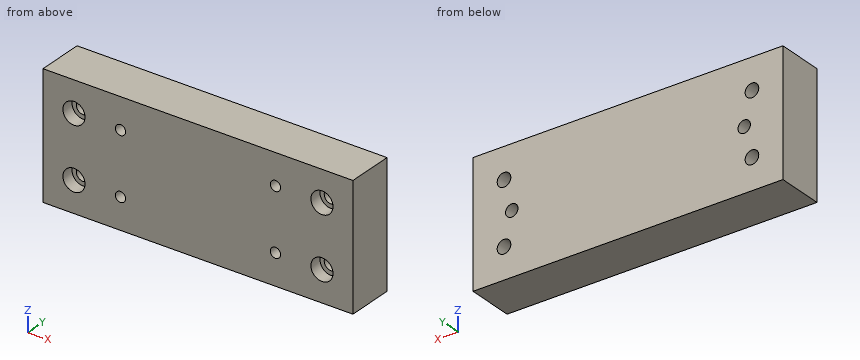
```python
from build123d import *

# Parameters (mm, degrees)
F0_W           = 200
F0_H           = 80
F1_DEPTH       = 30
F2_R           = 4
F3_DEPTH       = 10
F5_D           = 8.8
F5_CBORE_D     = 14.25
F5_CBORE_DEPTH = 8
F7_D           = 6.6
F7_DEPTH       = 12
F7_TIP         = 1.9828400428


with BuildPart() as f1:
    # F0 (on Front) → F1 (new body)
    with BuildSketch(Plane.XZ):
        Rectangle(F0_W, F0_H)
    extrude(amount=F1_DEPTH)

    # F2 (on face) → F3 (cut)
    with BuildSketch(Plane(origin=(0, 0, 0), x_dir=(-1, 0, 0), z_dir=(0, 1, 0))):
        with Locations((-75, 0)):
            Circle(F2_R)
        with Locations((75, 0)):
            Circle(F2_R)
    extrude(amount=-F3_DEPTH, mode=Mode.SUBTRACT)

    # F5 (through all)
    with Locations(Plane.XZ.offset(30)):
        with Locations((-80, 20), (-80, -20), (80, 20), (80, -20)):
            CounterBoreHole(F5_D / 2, F5_CBORE_D / 2, F5_CBORE_DEPTH)

    # F7
    with Locations(Plane.XZ.offset(30)):
        with Locations((-50, -20), (-50, 20), (50, 20), (50, -20)):
            Hole(F7_D / 2, depth=F7_DEPTH)
            with Locations((0, 0, -(F7_DEPTH + F7_TIP / 2))):  # 118° drill point
                Cone(0, F7_D / 2, F7_TIP, mode=Mode.SUBTRACT)


solid = f1.part
```
CAD build for the part. Positions are in the model's coordinates, mm. Round coordinates to 2 decimals unless told otherwise and drop trailing zeros. Order: outer loops, then holes, each group sorted by start corner. A loop starts at its lowest first (then second) coordinate and runs counter-clockwise, first axis right, second up.
Item 1: Probe line 1 along Z through (x, y) = (-80, -15.5); line 2 along Z through (x, y) = (80, -27.75) (3 decimals); line 3 along X through (y, z) = (-14, -16.5). List the from-to ranges inside material, lowest first.
Item 2: Saw through at B-B on z = 0. Write the cut outline in (x, y).
Item 3: Saw through at A-A on y = -8.25. Write the cut outline in (x, z).
Item 4: Pin check, flat tips, straight feed: pin 1 (4.5 mm diameter, centred on x = 79.5, z = -18.5, fed in from -Y) (1 decimal); pin 2 (4 mm diameter, centred on x = 76.5, z = 0.5, fed in from +Y); pin 3 (4.5 mm diameter, centred on x = -79.5, z = 23, fed in from -Y); pin 4 (5.5 mm diameter, centred on x = 50, z = 20, fed in from -Y). Stop position of each tip, or through.
Reported:
1. line 1: z = -40 to -24.4, -15.6 to 15.6, 24.4 to 40
1. line 2: z = -40 to -27.125, -12.875 to 12.875, 27.125 to 40
1. line 3: x = -100 to -82.67, -77.33 to 77.33, 82.67 to 100
2. outline: (-100, -30) - (100, -30) - (100, 0) - (79, 0) - (79, -10) - (71, -10) - (71, 0) - (-71, 0) - (-71, -10) - (-79, -10) - (-79, 0) - (-100, 0) - close
3. outline: (-100, -40) - (100, -40) - (100, 40) - (-100, 40) - close; hole circle Ø8.8 at (-80, -20); hole circle Ø8.8 at (-80, 20); hole circle Ø8 at (-75, 0); hole circle Ø8 at (75, 0); hole circle Ø8.8 at (80, -20); hole circle Ø8.8 at (80, 20)
4. pin 1: passes through
4. pin 2: stops at y = -10
4. pin 3: stops at y = -22
4. pin 4: stops at y = -17.67
